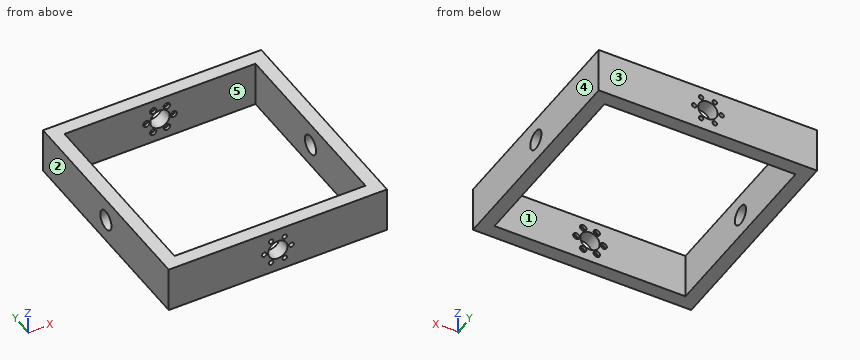
from build123d import *

# Parameters (mm, degrees)
BOSS_EXTRUDE1_DEPTH            = 76.2
BOSS_EXTRUDE1_DEPTH_BACK       = 76.2
SKETCH3_W                      = 152.4
SKETCH3_H                      = 152.4
SKETCH3_W_2                    = 133.35
SKETCH3_H_2                    = 133.35
SKETCH6_W                      = 152.4
SKETCH6_H                      = 120.65
CUT_EXTRUDE1_DEPTH             = 187.6511184
M12_CLEARANCE_HOLE1_D          = 13.5
M12_CLEARANCE_HOLE2_D          = 13.5
CBORE_FOR_M3_SHCS2_D           = 3.2
CBORE_FOR_M3_SHCS2_DEPTH       = 9.525
CBORE_FOR_M3_SHCS2_CBORE_D     = 4.5
CBORE_FOR_M3_SHCS2_CBORE_DEPTH = 2
CBORE_FOR_M3_SHCS3_D           = 3.2
CBORE_FOR_M3_SHCS3_DEPTH       = 9.525
CBORE_FOR_M3_SHCS3_CBORE_D     = 4.5
CBORE_FOR_M3_SHCS3_CBORE_DEPTH = 2


with BuildPart() as part:
    # Sketch3 → Boss-Extrude1 (new, two sides: drawn at the far end of the back side and taken through both)
    with BuildSketch(Plane.XY.offset(-BOSS_EXTRUDE1_DEPTH_BACK)):
        Rectangle(SKETCH3_W, SKETCH3_H)
        Rectangle(SKETCH3_W_2, SKETCH3_H_2, mode=Mode.SUBTRACT)
    extrude(amount=BOSS_EXTRUDE1_DEPTH + BOSS_EXTRUDE1_DEPTH_BACK)

    # Sketch6 → Cut-Extrude1 (cut, through all)
    with BuildSketch(Plane(origin=(0, 76.2, 0), x_dir=(1, 0, 0), z_dir=(0, 1, 0))):
        with Locations((0, 15.875)):
            Rectangle(SKETCH6_W, SKETCH6_H)
    extrude(amount=-CUT_EXTRUDE1_DEPTH, mode=Mode.SUBTRACT)

    # M12 Clearance Hole1 (through all)
    with Locations(Plane(origin=(0, 76.2, 0), x_dir=(1, 0, 0), z_dir=(0, 1, 0))):
        with Locations((0, -60.325)):
            Hole(M12_CLEARANCE_HOLE1_D / 2)

    # M12 Clearance Hole2 (through all)
    with Locations(Plane(origin=(76.2, 0, 0), x_dir=(0, 0, -1), z_dir=(1, 0, 0))):
        with Locations((-60.325, 0)):
            Hole(M12_CLEARANCE_HOLE2_D / 2)

    # CBORE for M3 SHCS2
    with Locations(Plane(origin=(0, 66.675, 0), x_dir=(-1, 0, 0), z_dir=(0, -1, 0))):
        with Locations((-4.7625, -68.573891971), (-4.7625, -52.076108029), (-9.525, -60.325), (9.525, -60.325), (4.7625, -52.076108029), (4.7625, -68.573891971)):
            CounterBoreHole(CBORE_FOR_M3_SHCS2_D / 2, CBORE_FOR_M3_SHCS2_CBORE_D / 2, CBORE_FOR_M3_SHCS2_CBORE_DEPTH, depth=CBORE_FOR_M3_SHCS2_DEPTH)

    # CBORE for M3 SHCS3
    with Locations(Plane(origin=(0, -66.675, 0), x_dir=(1, 0, 0), z_dir=(0, 1, 0))):
        with Locations((4.7625, -52.076108029), (9.525, -60.325), (4.7625, -68.664338764), (-4.7625, -68.664338764), (-9.525, -60.325), (-4.7625, -52.076108029)):
            CounterBoreHole(CBORE_FOR_M3_SHCS3_D / 2, CBORE_FOR_M3_SHCS3_CBORE_D / 2, CBORE_FOR_M3_SHCS3_CBORE_DEPTH, depth=CBORE_FOR_M3_SHCS3_DEPTH)


solid = part.part
CAD build for the part. Positions are in the model's coordinates, mm. Face numbers are marked on the shaded views. A direction names the side the tool comes from. Round coordinates to 2 decimals unless told otherwise and drop trailing zeros. Write each loop counter-clockwise with the first axis right and the second up, starting at its lowest first coordinate (ties: lowest second). Pieces come first, ordered by that corner, then holes.
(1) Mould opens along Y. For the marked faces 3, 4 and 5 say: pulls with the +Y half, pulls with the -Y half, needs draft (parallel to the pull), parting line crosses it, or undercut.
(2) Slice it at C-C, the plane x = 0. Write the cut outline in (y, z) (3 decimals).
(3) 3-axis set-ups, long thin cutter, end or side, ignore diameter. For the marked faces 1 and 2: which of +Z, -Z, +X, -X, +Y, -Y reach the whole face in a straight line?
(4) Probe line 1 along Y through (x, z) = (-41, 54) (3 decimals); line 2 along Z through (x, y) = (-8, -68.5). List the from-to ranges inside material, lowest first.
(5) Slice it at A-A, the plane y = -49. Write the cut outline in (x, z) (3 decimals), and give its area (3 significant figures).
From the geometry:
1. face 3: pulls with the +Y half
1. face 4: needs draft
1. face 5: undercut
2. outline: (-76.2, 44.45) - (-66.675, 44.45) - (-66.675, 53.575) - (-76.2, 53.575) - close; (-76.2, 67.075) - (-66.675, 67.075) - (-66.675, 76.2) - (-76.2, 76.2) - close; (66.675, 44.45) - (76.2, 44.45) - (76.2, 53.575) - (66.675, 53.575) - close; (66.675, 67.075) - (76.2, 67.075) - (76.2, 76.2) - (66.675, 76.2) - close
3. face 1: +Z, -Z
3. face 2: +Z, -Z, -X, +Y, -Y
4. line 1: y = -76.2 to -66.675, 66.675 to 76.2
4. line 2: z = 44.45 to 58.67, 61.98 to 76.2
5. outline: (-76.2, 44.45) - (-66.675, 44.45) - (-66.675, 76.2) - (-76.2, 76.2) - close; (66.675, 44.45) - (76.2, 44.45) - (76.2, 76.2) - (66.675, 76.2) - close
5. area: 605 mm2
